Autodesk Inventor part; units mm, degrees
ref_plane "YZ Plane" through (0, 0, 0) normal (1, 0, 0) x (0, 1, 0)
ref_plane "XZ Plane" through (0, 0, 0) normal (0, 1, 0) x (-1, 0, 0)
ref_plane "XY Plane" through (0, 0, 0) normal (0, 0, 1) x (1, 0, 0)
sketch "Sketch1" plane through (0, 0, 0) normal (0, 0, 1) x (1, 0, 0)
  line L0 (201.8785, 270.226) -> (-226.7465, -240.5894)
  line L1 (-226.7465, -240.5894) -> (-177.0105, -240.5894)
  line L2 (-177.0105, -240.5894) -> (201.8785, 210.9529)
  line L3 (201.8785, 210.9529) -> (201.8785, 270.226)
  line L4 (-12.434, 14.8183) -> (12.434, -14.8183) construction
  point P0 (0, 0)
  point P1 (0, 0)
  dimension "d0" = 50
  dimension "d1" = 38.1
  dimension "d2" = 428.625
extrude "Extrusion1" add sketch "Sketch1" along normal blind 9.525
sketch "Sketch2" plane through (0, 0, 9.525) normal (0, 0, 1) x (1, 0, 0)
  line L0 (201.8785, 210.9529) -> (201.8785, 270.226)
  line L1 (201.8785, 225.9981) -> (211.4035, 224.4106)
  line L2 (211.4035, 224.4106) -> (211.4035, 254.4106)
  line L3 (211.4035, 254.4106) -> (201.8785, 252.8231)
  line L4 (-226.7465, -240.5894) -> (-177.0105, -240.5894)
  point P0 (0, 0)
  point P1 (211.4035, 239.4106)
  dimension "d5" = 480
  dimension "d6" = 9.525
  dimension "d8" = 1.5875
  dimension "d9" = 30
extrude "Extrusion2" add sketch "Sketch2" against normal up to surface (9.525 mm away)
sketch "Sketch3" plane through (0, 0, 9.525) normal (0, 0, 1) x (1, 0, 0)
  circle A0 centre (0, 0) radius 12.7
  line L0 (201.8785, 270.226) -> (-226.7465, -240.5894)
  circle A1 centre (-24.4902, -29.1863) radius 12.7
  circle A2 centre (-48.9804, -58.3726) radius 12.7
  circle A3 centre (-73.4706, -87.5589) radius 12.7
  circle A4 centre (-97.9608, -116.7452) radius 12.7
  circle A5 centre (-122.451, -145.9315) radius 12.7
  circle A6 centre (-146.9412, -175.1178) radius 12.7
  circle A7 centre (-171.4315, -204.3041) radius 12.7
  circle A8 centre (24.4902, 29.1863) radius 12.7
  circle A9 centre (0, 0) radius 12.7
  circle A10 centre (-24.4902, -29.1863) radius 12.7
  circle A11 centre (-48.9804, -58.3726) radius 12.7
  circle A12 centre (-73.4706, -87.5589) radius 12.7
  circle A13 centre (-97.9608, -116.7452) radius 12.7
  circle A14 centre (-122.451, -145.9315) radius 12.7
  circle A15 centre (-146.9412, -175.1178) radius 12.7
  circle A16 centre (48.9804, 58.3726) radius 12.7
  circle A17 centre (24.4902, 29.1863) radius 12.7
  circle A18 centre (0, 0) radius 12.7
  circle A19 centre (-24.4902, -29.1863) radius 12.7
  circle A20 centre (-48.9804, -58.3726) radius 12.7
  circle A21 centre (-73.4706, -87.5589) radius 12.7
  circle A22 centre (-97.9608, -116.7452) radius 12.7
  circle A23 centre (-122.451, -145.9315) radius 12.7
  circle A24 centre (73.4706, 87.5589) radius 12.7
  circle A25 centre (48.9804, 58.3726) radius 12.7
  circle A26 centre (24.4902, 29.1863) radius 12.7
  circle A27 centre (0, 0) radius 12.7
  circle A28 centre (-24.4902, -29.1863) radius 12.7
  circle A29 centre (-48.9804, -58.3726) radius 12.7
  circle A30 centre (-73.4706, -87.5589) radius 12.7
  circle A31 centre (-97.9608, -116.7452) radius 12.7
  circle A32 centre (97.9608, 116.7452) radius 12.7
  circle A33 centre (73.4706, 87.5589) radius 12.7
  circle A34 centre (48.9804, 58.3726) radius 12.7
  circle A35 centre (24.4902, 29.1863) radius 12.7
  circle A36 centre (0, 0) radius 12.7
  circle A37 centre (-24.4902, -29.1863) radius 12.7
  circle A38 centre (-48.9804, -58.3726) radius 12.7
  circle A39 centre (-73.4706, -87.5589) radius 12.7
  circle A40 centre (122.451, 145.9315) radius 12.7
  circle A41 centre (97.9608, 116.7452) radius 12.7
  circle A42 centre (73.4706, 87.5589) radius 12.7
  circle A43 centre (48.9804, 58.3726) radius 12.7
  circle A44 centre (24.4902, 29.1863) radius 12.7
  circle A45 centre (0, 0) radius 12.7
  circle A46 centre (-24.4902, -29.1863) radius 12.7
  circle A47 centre (-48.9804, -58.3726) radius 12.7
  circle A48 centre (146.9412, 175.1178) radius 12.7
  circle A49 centre (122.451, 145.9315) radius 12.7
  circle A50 centre (97.9608, 116.7452) radius 12.7
  circle A51 centre (73.4706, 87.5589) radius 12.7
  circle A52 centre (48.9804, 58.3726) radius 12.7
  circle A53 centre (24.4902, 29.1863) radius 12.7
  circle A54 centre (0, 0) radius 12.7
  circle A55 centre (-24.4902, -29.1863) radius 12.7
  circle A56 centre (171.4315, 204.3041) radius 12.7
  circle A57 centre (146.9412, 175.1178) radius 12.7
  circle A58 centre (122.451, 145.9315) radius 12.7
  circle A59 centre (97.9608, 116.7452) radius 12.7
  circle A60 centre (73.4706, 87.5589) radius 12.7
  circle A61 centre (48.9804, 58.3726) radius 12.7
  circle A62 centre (24.4902, 29.1863) radius 12.7
  circle A63 centre (0, 0) radius 12.7
  dimension "d12" = 25.4
  dimension "d15" = 38.1
  dimension "d18" = 38.1
extrude "Extrusion3" cut sketch "Sketch3" against normal through all
chamfer "Chamfer1" distance 9.525 angle 11.388 1 edges at (-201.8785, -240.5894, 9.525) measured on face at (-210.1678, -240.5894, 3.175)
sketch "Sketch4" plane through (-226.7465, -240.5894, 0) normal (0, -0.9803, 0.1975) x (1, 0, 0)
  line L0 (33.5993, 0) -> (16.1368, 0)
  line L1 (16.1368, 0) -> (16.1368, 17.2439)
  line L2 (16.1368, 17.2439) -> (33.5993, 17.2439)
  line L3 (33.5993, 17.2439) -> (33.5993, 0)
  line L4 (51.3458, 9.7163) -> (1.6098, 9.7163)
  line L5 (51.3458, 9.7163) -> (428.625, 98.4954)
  line L6 (428.625, 98.4954) -> (428.625, 101.4661)
  line L7 (428.625, 101.4661) -> (438.15, 101.1527)
  line L8 (438.15, 101.1527) -> (438.15, 107.0762)
  line L9 (438.15, 107.0762) -> (428.625, 106.7628)
  line L10 (428.625, 106.7628) -> (428.625, 110.199)
  line L11 (428.625, 110.199) -> (1.6098, 9.7163)
  ellipse E0 centre (202.2563, 51.0795) end of major axis (214.9563, 51.0795) minor radius 2.5076
  ellipse E1 centre (128.7857, 33.7908) end of major axis (141.4857, 33.7908) minor radius 2.5076
  ellipse E2 centre (55.315, 16.5021) end of major axis (68.015, 16.5021) minor radius 2.5076
  ellipse E3 centre (79.8053, 22.265) end of major axis (92.5053, 22.265) minor radius 2.5076
  ellipse E4 centre (373.6878, 91.4197) end of major axis (386.3878, 91.4197) minor radius 2.5076
  ellipse E5 centre (251.2367, 62.6052) end of major axis (263.9367, 62.6052) minor radius 2.5076
  ellipse E6 centre (300.2171, 74.131) end of major axis (312.9171, 74.131) minor radius 2.5076
  ellipse E7 centre (177.7661, 45.3166) end of major axis (190.4661, 45.3166) minor radius 2.5076
  ellipse E8 centre (153.2759, 39.5537) end of major axis (165.9759, 39.5537) minor radius 2.5076
  ellipse E9 centre (275.7269, 68.3681) end of major axis (288.4269, 68.3681) minor radius 2.5076
  ellipse E10 centre (324.7073, 79.8939) end of major axis (337.4073, 79.8939) minor radius 2.5076
  ellipse E11 centre (226.7465, 56.8423) end of major axis (239.4465, 56.8423) minor radius 2.5076
  ellipse E12 centre (398.178, 97.1826) end of major axis (410.878, 97.1826) minor radius 2.5076
  ellipse E13 centre (104.2955, 28.0279) end of major axis (116.9955, 28.0279) minor radius 2.5076
  ellipse E14 centre (349.1975, 85.6568) end of major axis (361.8975, 85.6568) minor radius 2.5076
  line L12 (0, 0) -> (49.736, 0)
  point P0 (226.7465, 47.5049)
  point P1 (24.868, 0)
  point P2 (16.1368, 13.1347)
  dimension "d26" = 17.4625
extrude "Extrusion4" cut sketch "Sketch4" against normal blind 9.525 contours L0 L1 L4 L3 | L4 L1 L11 L3
equation "\"d8\" = 0.166667 * d6"
properties part number "SUPPORTS_TREBUCHET" material "Wood (Birch)"
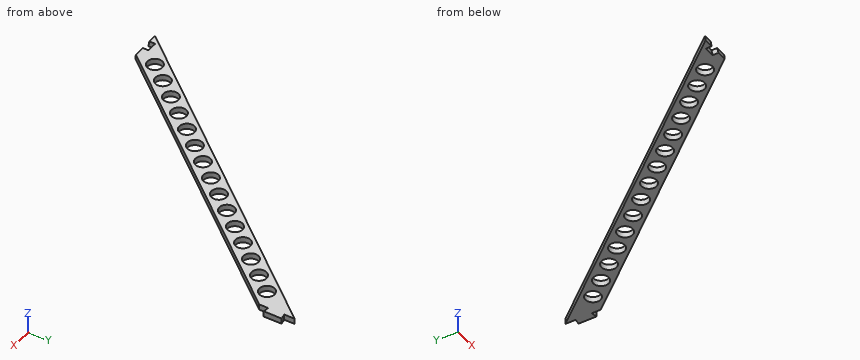
Model file for the job. Use its own axes, mm. Give positions to 0.01 mm unless a question says otherwise; leave off trailing zeros. Write each loop counter-clockwise with the first axis right and the second up, starting at its lowest first coordinate (ties: lowest second). Pieces come first, ordered by that corner, then holes. Notation, with made-up numbers: M 52,3 L 84,3 A24 ccw 84,42 Z; hole C 56,51.25 d7. An arc over 180 degrees is marked long. One line per item, written item: value. Start each with the question number.
Q1. Saw through at C-C, the plane y = 0. Write the cut outline in (x, z) (3 decimals).
Q2. Saw through at A-A, the plane x = -124.5. Write the cut outline in (y, z) (3 decimals).
Q3. Probe probe 1 along Y at (x, z) = (-26, 8.75); probe 2 along X at (y, z) = (-200, 5.5); probe 3 along Y at (x, z) = (34.5, 4.75). List the from-to ranges inside material, lowest first. Write a range as [from, to].
Q4. Drop flat-ended pins along their axis: pin 1 Ø3 at (y, z) = (-23.5, 5.5) entering from -X; pin 2 Ø5 at (y, z) = (48.5, 6.5) entering from -X; pin 3 Ø3 at (y, z) = (57, 6) entering from +X. Give the stop position or say it passes through.
Q5. Saw through at B-B, the plane z = 4. State how many separate pieces and enclosed holes the cut face has, plus the area to 3 significant figures.
Output values:
1. outline: M -24.868,0 L -12.7,0 L -12.7,9.525 L -24.868,9.525 Z; M 12.7,0 L 24.868,0 L 24.868,9.525 L 12.7,9.525 Z
2. outline: M -178.01,0 L -158.465,0 L -158.465,9.525 L -178.01,9.525 Z; M -133.398,0 L -118.737,0 L -118.737,9.525 L -133.398,9.525 Z
3. probe 1: y = [-60.62, -41.8], [-16.58, -1.35]
3. probe 2: x = [-192.69, -183.38], [-159.48, -142.95]
3. probe 3: y = [11.48, 21.37], [37, 70.75]
4. pin 1: stops at x = -45.85
4. pin 2: stops at x = 13.73
4. pin 3: stops at x = 73.96
5. separate pieces: 1
5. enclosed holes: 15
5. area: 16,400 mm²
